```python
from build123d import *

# Parameters (mm, degrees)
SKETCH1_W           = 57.15
SKETCH1_H           = 152.4
BOSS_EXTRUDE1_DEPTH = 3.175
SKETCH2_W           = 4.195
SKETCH2_H           = 6.35
SKETCH2_W_2         = 7.37
CUT_EXTRUDE1_DEPTH  = 4.175


with BuildPart() as part:
    # Sketch1 → Boss-Extrude1 (new body)
    with BuildSketch(Plane(origin=(0, 0, 0), x_dir=(1, 0, 0), z_dir=(0, 1, 0))):
        Rectangle(SKETCH1_W, SKETCH1_H)
    extrude(amount=BOSS_EXTRUDE1_DEPTH)

    # Sketch2 → Cut-Extrude1 (cut, through all)
    with BuildSketch(Plane(origin=(0, 3.175, 0), x_dir=(1, 0, 0), z_dir=(0, 1, 0))):
        with Locations((-26.4775, -73.025)):
            Rectangle(SKETCH2_W, SKETCH2_H)
        with Locations((-3.685, -73.025)):
            Rectangle(SKETCH2_W_2, SKETCH2_H)
        with Locations((3.685, -73.025)):
            Rectangle(SKETCH2_W_2, SKETCH2_H)
        with Locations((26.4775, -73.025)):
            Rectangle(SKETCH2_W, SKETCH2_H)
    cut_extrude1 = extrude(amount=-CUT_EXTRUDE1_DEPTH, mode=Mode.SUBTRACT)

    # Mirror1: Cut-Extrude1 across plane
    add(cut_extrude1.mirror(Plane.XY), mode=Mode.SUBTRACT)


solid = part.part
```
For this review, take the finished solid that the model builds, in its own axes (mm). A direction names the side the tool comes from. Give positions to 0.01 mm unless a question says otherwise; leave off trailing zeros. Order: outer loops, then holes, each group sorted by start corner. A loop starts at its lowest first (then second) coordinate and runs counter-clockwise, first axis right, second up.
1) The part is to be moulded in two halves that separate along X. For faces 1 (the face through (0, 0, -1)), 2 (the face through (-7.37, 2, -73)), 3 (the face through (24.38, 2, -73)), 4 (the face through (-24.38, 2, -73)), say which applies: released by +X, released by -X, zero draft, split by the parting line, or undercut.
2) Insertion check: pin 1 (1 mm diameter, centred on x = 3, y = 1.5, fed in from -Z); pin 2 (1.6 mm diameter, centred on y = 1, z = -73.5, fed in from +X); pin 3 (1 mm diameter, centred on y = 2, z = -72.5, fed in from -X). Each pin has a flat end and moves straight along its axis. Give the tip position at first contact, or say it passes through.
3) Take a section at A-A (y = 0.75). Give the boundary of the cut face in (x, z) (3 decimals), then the cut area to 3 significant figures.
4) Wall thickness on line 1 (Z direction, x = 5, y = 2): over which ranges is the line inside the solid? List them lowest first.
5) For faces 5 (the face through (-7.37, 2, 73)), 6 (the face through (26, 2, 69.85)), 7 (the face through (-27, 2, -69.85)), 8 (the face through (-24.38, 2, 73)), list the 3-axis set-ups (+Z, -Z, +X, -X, +Y, -Y) from which the entire face can be reached by the end or side of a thin tool; tool diameter is ignored.
Derived:
1. face 1: zero draft
1. face 2: undercut
1. face 3: released by +X
1. face 4: released by -X
2. pin 1: stops at z = -69.85
2. pin 2: stops at x = 24.38
2. pin 3: stops at x = -24.38
3. outline: (-28.575, -69.85) - (-24.38, -69.85) - (-24.38, -76.2) - (-7.37, -76.2) - (-7.37, -69.85) - (7.37, -69.85) - (7.37, -76.2) - (24.38, -76.2) - (24.38, -69.85) - (28.575, -69.85) - (28.575, 69.85) - (24.38, 69.85) - (24.38, 76.2) - (7.37, 76.2) - (7.37, 69.85) - (-7.37, 69.85) - (-7.37, 76.2) - (-24.38, 76.2) - (-24.38, 69.85) - (-28.575, 69.85) - close
3. area: 8,420 mm2
4. line 1: z = -69.85 to 69.85
5. face 5: +Z, +Y, -Y
5. face 6: +Z, +X, +Y, -Y
5. face 7: -Z, -X, +Y, -Y
5. face 8: +Z, -X, +Y, -Y
